CAD build for the part. Positions are in the model's coordinates, mm. Round coordinates to 2 decimals unless told otherwise and drop trailing zeros. Loops run counter-clockwise (first coordinate to the right, second up) from the corner with the lowest first, then second, coordinate; pieces in that order, holes last. Notation, with made-up numbers: (76.25, 87.5) -> (122.25, 87.5) arc R34 cw to (122.25, 126.5) -> close; hole circle Ø11 at (63, 88). An arc over 180 degrees is marked (long way). Answer as CSV lines item,"result".
```python
from build123d import *

# Parameters (mm, degrees)
SKETCH1_R                        = 25.4
BOSS_EXTRUDE1_DEPTH              = 20
SKETCH2_R                        = 16
CUT_EXTRUDE1_DEPTH               = 21
F_10_5_10_5_DIAMETER_HOLE1_D     = 10.5
F_10_5_10_5_DIAMETER_HOLE1_DEPTH = 30
F_10_5_10_5_DIAMETER_HOLE1_TIP   = 3.15451825


with BuildPart() as part:
    # Sketch1 → Boss-Extrude1 (new body)
    with BuildSketch(Plane(origin=(0, 0, 0), x_dir=(1, 0, 0), z_dir=(0, 1, 0))):
        Circle(SKETCH1_R)
    extrude(amount=BOSS_EXTRUDE1_DEPTH)

    # Sketch2 → Cut-Extrude1 (cut, through all)
    with BuildSketch(Plane(origin=(0, 20, 0), x_dir=(1, 0, 0), z_dir=(0, 1, 0))):
        Circle(SKETCH2_R)
    extrude(amount=-CUT_EXTRUDE1_DEPTH, mode=Mode.SUBTRACT)

    # Ø10.5 (10.5) Diameter Hole1
    with Locations(Plane(origin=(-6.456859903, 10, -24.565605228), x_dir=(-0.967149812, 0, 0.254207083), z_dir=(-0.254207083, 0, -0.967149812))):
        with Locations((0, 0)):
            Hole(F_10_5_10_5_DIAMETER_HOLE1_D / 2, depth=F_10_5_10_5_DIAMETER_HOLE1_DEPTH)
            with Locations((0, 0, -(F_10_5_10_5_DIAMETER_HOLE1_DEPTH + F_10_5_10_5_DIAMETER_HOLE1_TIP / 2))):  # 118° drill point
                Cone(0, F_10_5_10_5_DIAMETER_HOLE1_D / 2, F_10_5_10_5_DIAMETER_HOLE1_TIP, mode=Mode.SUBTRACT)


solid = part.part
```
Q1. Slice it at D-D, the plane y = 12.25. Give the cut face in (x, z).
Results:
outline,"(-10.93, -22.93) -> (-8.47, -13.57) arc R16 cw (long way) to (0.7, -15.98) -> (-1.76, -25.34) arc R25.4 ccw (long way) to start"
Q2. Slice it at A-A, the plane z = 8. Give the cut face in (x, y), and give its area (3 significant figures).
Results:
outline,"(-24.11, 0) -> (-13.86, 0) -> (-13.86, 20) -> (-24.11, 20) -> close; (13.86, 0) -> (24.11, 0) -> (24.11, 20) -> (13.86, 20) -> close"
area,"410 mm2"
Q3. Drop flat-ended pins along their axis: pin 1 Ø1 at (y, z) = (7.5, -7) entering from -X; pin 2 Ø1 at (y, z) = (8, -17.5) entering from -X; pin 3 Ø12 at (x, y) = (-3, 14) entering from -Z. Give the stop position or say it passes through.
Results:
pin 1,"x = -24.55"
pin 2,"x = -18.87"
pin 3,"z = -25.4"
Q4. Two-plate mould, pull along Z, no slides. Class faces 1 (the cylindrical face through (-3.47, 10.14, 15.62)), 2 (the flat face through (0, 20, 17)), 3 (the cylindrical face through (-5.506, 9.86, 24.796)): pulls with the +Z half, pulls with the -Z half, needs draft (parallel to the pull), parting line crosses it, or undercut.
Results:
face 1,"undercut"
face 2,"needs draft"
face 3,"parting line crosses it"
Q5. Slice it at B-B, the plane x = 6.5. Give the cut face in (y, z), and give its area (3 significant figures).
Results:
outline,"(0, -24.55) -> (20, -24.55) -> (20, -14.62) -> (0, -14.62) -> close; (0, 14.62) -> (20, 14.62) -> (20, 24.55) -> (0, 24.55) -> close"
area,"397 mm2"
Q6. Probe L1, parallel to X at y = 7.5, z = 0; L2, parallel to Z at x = 3, y = 11.25. List the from-to ranges inside material, lowest first. Write a range as [from, to].
Results:
L1,"[-25.4, -16], [16, 25.4]"
L2,"[-25.22, -15.72], [15.72, 25.22]"
Q7. Slice it at C-C, the plane y = 18.75. Give the cut face in (x, z).
Results:
outline,"circle Ø50.8 at (0, 0); hole circle Ø32 at (0, 0)"
